For this review, take the finished solid that the model builds, in its own axes (mm). A direction names the side the tool comes from. Coordinates: 2 decimals unless noted, no trailing zeros. Loops run counter-clockwise (first coordinate to the right, second up) from the corner with the lowest first, then second, coordinate; pieces in that order, holes last. Notation, with made-up numbers: (-17, 18.5) - (-7, 18.5) arc R20 ccw to (-7, 40.5) - close; hole circle Ø6 at (-3.75, 50.25). An arc over 180 degrees is marked (long way). One line per item, written item: value. Start each with the question number.
1. The part is to be moulded in two halves that separate along X. For faces 3 (the face through (38.1, 7, 3)), 4 (the face through (254, 50, 3)), 5 (the face through (1.27, 8, 3)), say which applies: released by +X, released by -X, zero draft, split by the parting line, or undercut.
2. For faces 1 (the face through (126, 101.016, 3)), 2 (the face through (34, 3.454, 3)), list the 3-axis set-ups (+Z, -Z, +X, -X, +Y, -Y) from which the entire face can be reached by the end or side of a thin tool; tool diameter is ignored.
3. Insertion check: pin 1 (3 mm diameter, centred on y = 10, z = 4, fed in from -X). The pin has a flat end and moves straight along its axis. Give the tip position at first contact, or say it passes through.
4. To check wall thickness, follow line 1 (Y direction, x = 136.5, z = 2.55); line 2 (Y direction, x = 65, z = 5.8); line 3 (X direction, y = 24.5, z = 0.8). State the ranges of each line that lie inside material, in increasing order. Write a range as from..to.
5. Take a section at B-B, the plane z = 2. Count the separate pieces of the cut face and the enclosed holes in it, and give its area (3 significant figures).
6. Take a section at A-A, the plane y = 43.5. State the section outline as (x, z) points.
```python
from build123d import *

# Parameters (mm, degrees)
SKETCH1_W           = 254
SKETCH1_H           = 101.0158
SKETCH1_W_2         = 6.35
SKETCH1_H_2         = 7.62
BOSS_EXTRUDE1_DEPTH = 6
SKETCH2_R           = 1.778
CUT_EXTRUDE1_DEPTH  = 274.415785663
SKETCH3_W           = 7.62
SKETCH3_H           = 6
CUT_EXTRUDE2_DEPTH  = 274.415785663
CUT_EXTRUDE3_REACH  = 275.416
SKETCH4_W           = 7.62
SKETCH4_H           = 0.35
SKETCH8_W           = 1.27
SKETCH8_H           = 12.7
CUT_EXTRUDE6_DEPTH  = 274.415785663
FILLET1_R           = 2.54
SKETCH6_R           = 1.8034
CUT_EXTRUDE4_DEPTH  = 274.415785663
SKETCH7_R           = 1.5875
CUT_EXTRUDE5_DEPTH  = 274.415785663


with BuildPart() as part:
    # Sketch1 → Boss-Extrude1 (new body)
    with BuildSketch(Plane.XY):
        with Locations((127, 50.5079)):
            Rectangle(SKETCH1_W, SKETCH1_H)
        with Locations((225.425, 93.7514)):
            Rectangle(SKETCH1_W_2, SKETCH1_H_2, mode=Mode.SUBTRACT)
        with Locations((66.675, 93.7514)):
            Rectangle(SKETCH1_W_2, SKETCH1_H_2, mode=Mode.SUBTRACT)
        with Locations((225.425, 7.2644)):
            Rectangle(SKETCH1_W_2, SKETCH1_H_2, mode=Mode.SUBTRACT)
        with Locations((66.675, 7.2644)):
            Rectangle(SKETCH1_W_2, SKETCH1_H_2, mode=Mode.SUBTRACT)
    extrude(amount=BOSS_EXTRUDE1_DEPTH)

    # Sketch2 → Cut-Extrude1 (cut, through all)
    with BuildSketch(Plane.XY.offset(6)):
        with Locations((241.3, 52.2605)):
            Circle(SKETCH2_R)
        with BuildLine():
            Line((16.51, 70.307310217), (19.05, 70.307310217))
            ThreePointArc((19.05, 70.307310217), (20.6375, 68.719810217), (19.05, 67.132310217))
            Line((19.05, 67.132310217), (16.51, 67.132310217))
            ThreePointArc((16.51, 67.132310217), (14.9225, 68.719810217), (16.51, 70.307310217))
        make_face()
        with BuildLine():
            Line((16.51, 26.466689783), (19.05, 26.466689783))
            ThreePointArc((19.05, 26.466689783), (20.6375, 24.879189783), (19.05, 23.291689783))
            Line((19.05, 23.291689783), (16.51, 23.291689783))
            ThreePointArc((16.51, 23.291689783), (14.9225, 24.879189783), (16.51, 26.466689783))
        make_face()
        with BuildLine():
            Line((16.51, 58.0495), (19.05, 58.0495))
            ThreePointArc((19.05, 58.0495), (30.3, 46.7995), (19.05, 35.5495))
            Line((19.05, 35.5495), (16.51, 35.5495))
            ThreePointArc((16.51, 35.5495), (5.26, 46.7995), (16.51, 58.0495))
        make_face()
    extrude(amount=-CUT_EXTRUDE1_DEPTH, mode=Mode.SUBTRACT)

    # Sketch3 → Cut-Extrude2 (cut, through all)
    with BuildSketch(Plane.XY.offset(6)):
        with Locations((34.29, 94.5614)):
            Rectangle(SKETCH3_W, SKETCH3_H)
        with Locations((148.59, 94.5614)):
            Rectangle(SKETCH3_W, SKETCH3_H)
        with Locations((148.59, 6.4544)):
            Rectangle(SKETCH3_W, SKETCH3_H)
        with Locations((34.29, 6.4544)):
            Rectangle(SKETCH3_W, SKETCH3_H)
    extrude(amount=-CUT_EXTRUDE2_DEPTH, mode=Mode.SUBTRACT)

    # Sketch4 → Cut-Extrude3 (cut, up to next)
    with BuildSketch(Plane.XY.offset(6), mode=Mode.PRIVATE) as cut_extrude3_sk1:
        with Locations((34.29, 91.3864)):
            Rectangle(SKETCH4_W, SKETCH4_H)
    cut_extrude3_tool1 = extrude(cut_extrude3_sk1.sketch, amount=-CUT_EXTRUDE3_REACH, mode=Mode.PRIVATE) & part.part
    # Sketch4 → Cut-Extrude3 (cut, up to next)
    with BuildSketch(Plane.XY.offset(6), mode=Mode.PRIVATE) as cut_extrude3_sk2:
        with Locations((34.29, 9.6294)):
            Rectangle(SKETCH4_W, SKETCH4_H)
    cut_extrude3_tool2 = extrude(cut_extrude3_sk2.sketch, amount=-CUT_EXTRUDE3_REACH, mode=Mode.PRIVATE) & part.part
    # Sketch4 → Cut-Extrude3 (cut, up to next)
    with BuildSketch(Plane.XY.offset(6), mode=Mode.PRIVATE) as cut_extrude3_sk3:
        with Locations((148.59, 91.3864)):
            Rectangle(SKETCH4_W, SKETCH4_H)
    cut_extrude3_tool3 = extrude(cut_extrude3_sk3.sketch, amount=-CUT_EXTRUDE3_REACH, mode=Mode.PRIVATE) & part.part
    # Sketch4 → Cut-Extrude3 (cut, up to next)
    with BuildSketch(Plane.XY.offset(6), mode=Mode.PRIVATE) as cut_extrude3_sk4:
        with Locations((148.59, 9.6294)):
            Rectangle(SKETCH4_W, SKETCH4_H)
    cut_extrude3_tool4 = extrude(cut_extrude3_sk4.sketch, amount=-CUT_EXTRUDE3_REACH, mode=Mode.PRIVATE) & part.part
    add(cut_extrude3_tool1.solids().sort_by_distance((34.29, 91.3864, 6))[0], mode=Mode.SUBTRACT)
    add(cut_extrude3_tool2.solids().sort_by_distance((34.29, 9.6294, 6))[0], mode=Mode.SUBTRACT)
    add(cut_extrude3_tool3.solids().sort_by_distance((148.59, 91.3864, 6))[0], mode=Mode.SUBTRACT)
    add(cut_extrude3_tool4.solids().sort_by_distance((148.59, 9.6294, 6))[0], mode=Mode.SUBTRACT)

    # Sketch8 → Cut-Extrude6 (cut, through all)
    with BuildSketch(Plane.XY.offset(6)):
        with Locations((0.635, 94.6658)):
            Rectangle(SKETCH8_W, SKETCH8_H)
        with Locations((0.635, 6.35)):
            Rectangle(SKETCH8_W, SKETCH8_H)
    extrude(amount=-CUT_EXTRUDE6_DEPTH, mode=Mode.SUBTRACT)

    # Fillet1
    # the kernel refuses this fillet: 2.54 mm, written as the material it takes off along each edge
    with BuildSketch(Plane(origin=(254, 0, -6.35), x_dir=(-1, 0, 0), z_dir=(0, 0, 1)), Plane(origin=(254, 101.0158, -6.35), x_dir=(0, -1, 0), z_dir=(0, 0, 1)), Plane(origin=(1.27, 0, 12.35), x_dir=(1, 0, 0), z_dir=(0, 0, -1)), Plane(origin=(1.27, 101.0158, 12.35), x_dir=(0, -1, 0), z_dir=(0, 0, -1))) as fillet1_piece_1:
        with BuildLine():
            CenterArc((FILLET1_R, -FILLET1_R), FILLET1_R, 90, 90)
            Line((0, -FILLET1_R), (-FILLET1_R * 0.02, -FILLET1_R))
            Line((-FILLET1_R * 0.02, -FILLET1_R), (-FILLET1_R * 0.02, FILLET1_R * 0.02))
            Line((-FILLET1_R * 0.02, FILLET1_R * 0.02), (FILLET1_R, FILLET1_R * 0.02))
            Line((FILLET1_R, FILLET1_R * 0.02), (FILLET1_R, 0))
        make_face()
    extrude(amount=18.7, mode=Mode.SUBTRACT)
    with BuildSketch(Plane(origin=(0, 88.3158, 11.499261314), x_dir=(0, -1, 0), z_dir=(0, 0, -1))) as fillet1_piece_2:
        with BuildLine():
            CenterArc((2.199704526, -2.54), FILLET1_R, 90, 60)
            Line((0, -1.27), (-0.043994091, -1.2446))
            ThreePointArc((-0.043994091, -1.2446), (-0.0508, -0.635), (-0.0508, 0))
            Line((-0.0508, 0), (0, 0.0508))
            Line((0, 0.0508), (2.199704526, 0.0508))
            Line((2.199704526, 0.0508), (2.199704526, 0))
        make_face()
    extrude(amount=16.998522628, mode=Mode.SUBTRACT)
    with BuildSketch(Plane(origin=(0, 12.7, 11.499261314), x_dir=(1, 0, 0), z_dir=(0, 0, -1))) as fillet1_piece_3:
        with BuildLine():
            CenterArc((2.54, -2.199704526), FILLET1_R, 120, 60)
            Line((0, -2.199704526), (-0.0508, -2.199704526))
            Line((-0.0508, -2.199704526), (-0.0508, 0))
            Line((-0.0508, 0), (0, 0.0508))
            ThreePointArc((0, 0.0508), (0.635, 0.0508), (1.2446, 0.043994091))
            Line((1.2446, 0.043994091), (1.27, 0))
        make_face()
    extrude(amount=16.998522628, mode=Mode.SUBTRACT)

    # Sketch6 → Cut-Extrude4 (cut, through all)
    with BuildSketch(Plane.XY.offset(6)):
        with Locations((46.0121, 6.4544)):
            Circle(SKETCH6_R)
        with Locations((136.8679, 6.4544)):
            Circle(SKETCH6_R)
        with Locations((46.0121, 94.5614)):
            Circle(SKETCH6_R)
        with Locations((136.8679, 94.5614)):
            Circle(SKETCH6_R)
    extrude(amount=-CUT_EXTRUDE4_DEPTH, mode=Mode.SUBTRACT)

    # Sketch7 → Cut-Extrude5 (cut, through all)
    with BuildSketch(Plane.XY.offset(6)):
        with Locations((241.3, 0)):
            Circle(SKETCH7_R)
    extrude(amount=-CUT_EXTRUDE5_DEPTH, mode=Mode.SUBTRACT)


solid = part.part
```
Solutions:
1. face 3: undercut
1. face 4: released by +X
1. face 5: released by -X
2. face 1: +Z, -Z, +X, -X, +Y
2. face 2: +Z, -Z
3. pin 1: x = 1.27
4. line 1: 0..4.69, 8.22..92.8, 96.33..101.02
4. line 2: 0..3.45, 11.07..89.94, 97.56..101.02
4. line 3: 0..14.97, 20.59..254
5. separate pieces: 1
5. enclosed holes: 16
5. area: 24,700 mm2
6. outline: (0, 0) - (5.75, 0) - (5.75, 6) - (0, 6) - close; (29.81, 0) - (254, 0) - (254, 6) - (29.81, 6) - close
